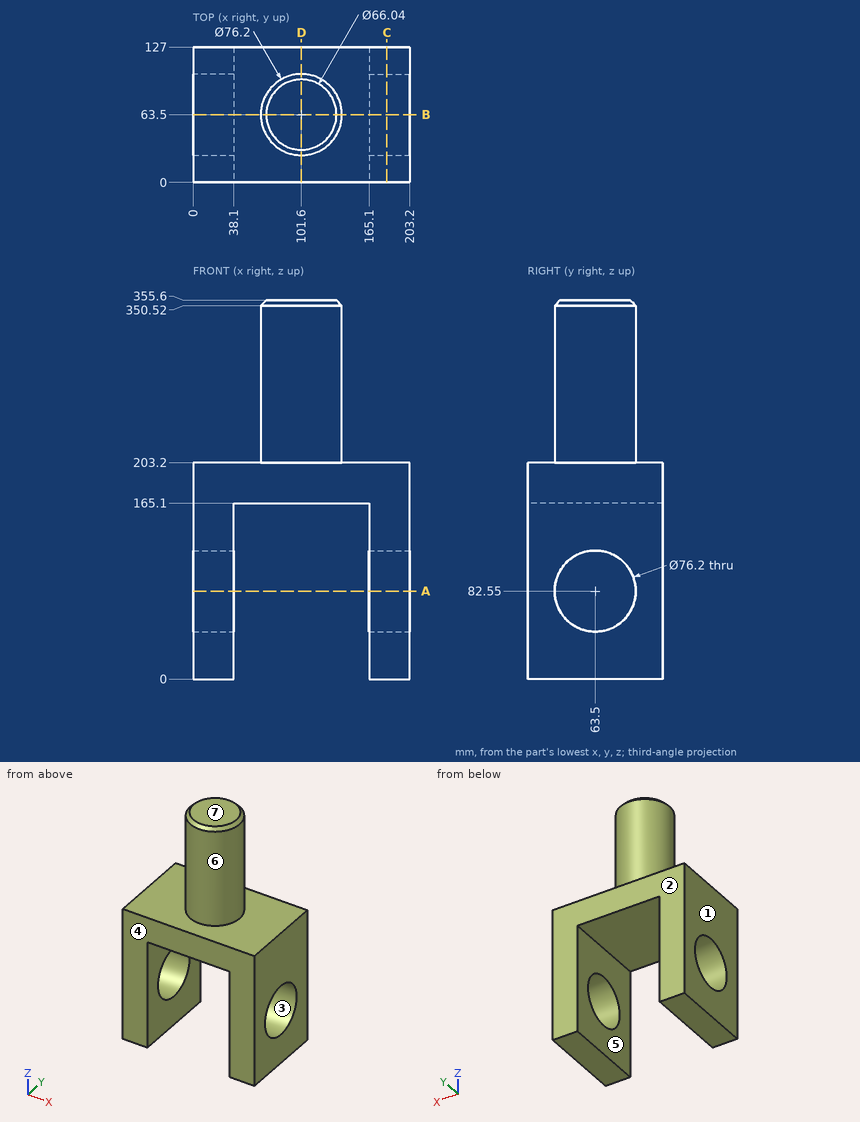
Design review of the part shown in the three views and the two pictorial views. Dimensions are in mm from the part's minimum x, y and z. A direction names the side the tool comes from. Coordinates: 2 decimals unless noted, no trailing zeros. Write each loop counter-clockwise with the first axis right and the second up, starting at its lowest first coordinate (ties: lowest second). Pieces come first, ordered by that corner, then holes.
1) To check wall thickness, follow probe 1 along X at (y, z) = (26, 44.5); probe 2 along Y at (x, z) = (22, 82); probe 3 along Z at (x, y) = (185, 63). State the ranges of each line that lie inside material, in increasing order.
2) The part is to be moulded in two halves that separate along Y. For the marked faces 1, 2, 3 and 4, say which applies: pulls with the +Y half, pulls with the -Y half, needs draft (parallel to the pull), parting line crosses it, or undercut.
3) We need section A-A on z = 82.55. State the section outline as (x, y) points, then the cut area to 3 significant figures.
4) Machinability: for the marked faces 5, 6 and 7, which of the approach directions +Z, -Z, +X, -X, +Y, -Y give a long, thin tool a straight path to every point of the face, cutting with its end or side? Answer none if there is none.
5) We need section D-D on x = 101.6. State the section outline as (y, z) points.
6) Clearance check with flat-ended pins moving along their axes: pin 1 Ø6 at (x, y) = (60, 13.5) entering from +Z; pin 2 Ø4 at (x, y) = (135.5, 103.5) entering from -Z. State where each tip first meets the part, or that it passes through.
7) We need section B-B on y = 63.5. State the section outline as (x, z) points, then the cut area to 3 significant figures.
8) We need section C-C on x = 182. State the section outline as (y, z) points.
Answer list:
1. probe 1: x = 0 to 38.1, 165.1 to 203.2
1. probe 2: y = 0 to 25.4, 101.6 to 127
1. probe 3: z = 0 to 44.45, 120.65 to 203.2
2. face 1: needs draft
2. face 2: pulls with the +Y half
2. face 3: undercut
2. face 4: pulls with the -Y half
3. outline: (0, 0) - (38.1, 0) - (38.1, 25.4) - (0, 25.4) - close; (0, 101.6) - (38.1, 101.6) - (38.1, 127) - (0, 127) - close; (165.1, 0) - (203.2, 0) - (203.2, 25.4) - (165.1, 25.4) - close; (165.1, 101.6) - (203.2, 101.6) - (203.2, 127) - (165.1, 127) - close
3. area: 3,870 mm2
4. face 5: -Z, +Y, -Y
4. face 6: +Z
4. face 7: +Z, +X, -X, +Y, -Y
5. outline: (0, 165.1) - (127, 165.1) - (127, 203.2) - (101.6, 203.2) - (101.6, 350.52) - (96.52, 355.6) - (30.48, 355.6) - (25.4, 350.52) - (25.4, 203.2) - (0, 203.2) - close
6. pin 1: stops at z = 203.2
6. pin 2: stops at z = 165.1
7. outline: (0, 0) - (38.1, 0) - (38.1, 44.45) - (0, 44.45) - close; (0, 120.65) - (38.1, 120.65) - (38.1, 165.1) - (165.1, 165.1) - (165.1, 120.65) - (203.2, 120.65) - (203.2, 203.2) - (139.7, 203.2) - (139.7, 350.52) - (134.62, 355.6) - (68.58, 355.6) - (63.5, 350.52) - (63.5, 203.2) - (0, 203.2) - close; (165.1, 0) - (203.2, 0) - (203.2, 44.45) - (165.1, 44.45) - close
7. area: 26,100 mm2
8. outline: (0, 0) - (127, 0) - (127, 203.2) - (0, 203.2) - close; hole circle Ø76.2 at (63.5, 82.55)
